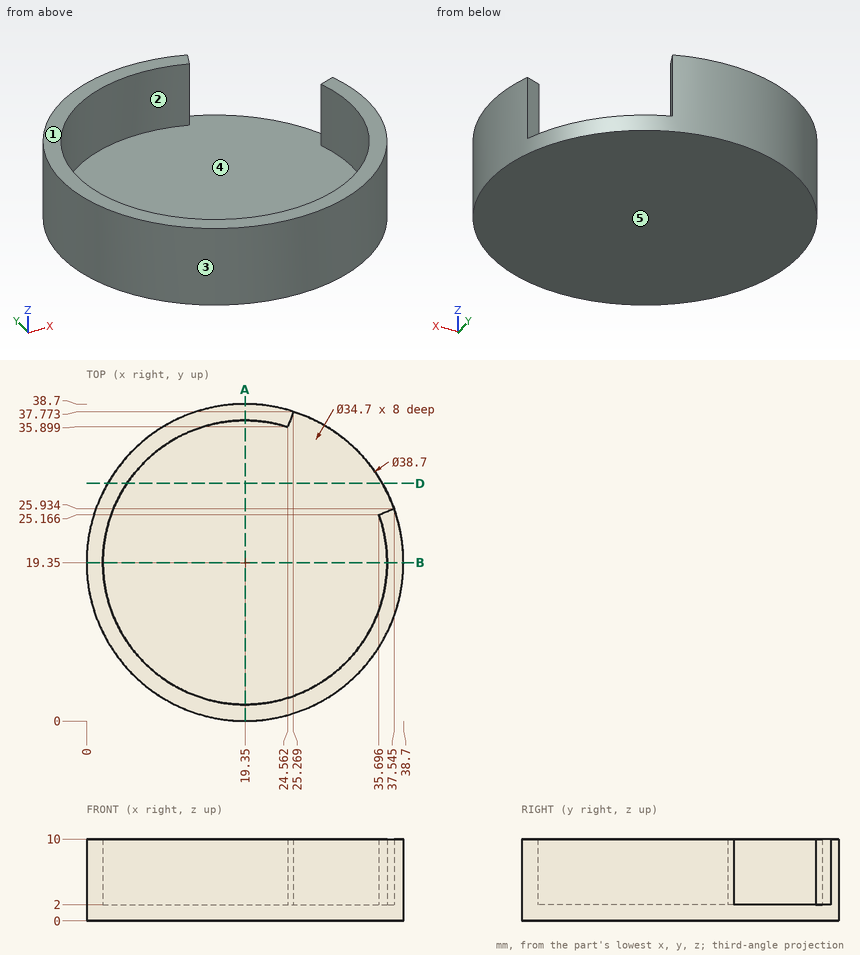
Could you check a few things on this drawing? It's one solid part, dimensions in mm from its lowest x, y, z. A direction names the side the tool comes from. Round coordinates to 2 decimals unless told otherwise and drop trailing zeros. Write each loop counter-clockwise with the first axis right and the second up, starting at its lowest first coordinate (ties: lowest second). Pieces come first, ordered by that corner, then holes.
Q1. If we mould it in two halves opening along Y, with no side actions, what happens to the marked faces 1, 2 and 3? For each: +Y half, -Y half, draft (parallel to the pull), parting line (faces both ways), or undercut.
Q2. Will these pins go through, and if not, where does the flat tip stop? P1, Ø1.5, axis at y = 15, z = 5.5, coming from the -X side; P2, Ø3, axis at x = 8, z = 7.5, coming from the +Y side (1 decimal); P3, Ø2, axis at x = 28.5, z = 6, coming from the +Y side.
Q3. Which directions (+Z, -Z, +X, -X, +Y, -Y) give clear straight access to the entire face, cutting with the end or side of a thin tool? Please do the marked faces 4 and 5.
Q4. If we section it at D-D on y = 29: Write out the boundary of the cut face in (x, z).
Q5. Please list where these lines run through material, in increasing order: probe 1 along X at (y, z) = (19.35, 6.25); probe 2 along Z at (x, y) = (27, 34).
Q6. If we section it at A-A on x = 19.35: Write out the boundary of the cut face in (y, z).
Answer below:
1. face 1: draft
1. face 2: undercut
1. face 3: parting line
2. P1: stops at x = 0.34
2. P2: stops at y = 36
2. P3: stops at y = 5.28
3. face 4: +Z
3. face 5: -Z, +X, -X, +Y, -Y
4. outline: (2.58, 0) - (36.12, 0) - (36.12, 2) - (4.93, 2) - (4.93, 10) - (2.58, 10) - close
5. probe 1: x = 0 to 2, 36.7 to 38.7
5. probe 2: z = 0 to 2
6. outline: (0, 0) - (38.7, 0) - (38.7, 10) - (36.7, 10) - (36.7, 2) - (2, 2) - (2, 10) - (0, 10) - close
